For this review, take the finished solid that the model builds, in its own axes (mm). Face numbers are marked on the shaded views. Give positions to 0.01 mm unless a question says otherwise; leave off trailing zeros. Loops run counter-clockwise (first coordinate to the right, second up) from the corner with the lowest first, then second, coordinate; pieces in that order, holes last. Notation, with made-up numbers: (79.25, 2) - (101.25, 2) arc R23 ccw to (101.25, 27) - close; hole circle Ø5 at (58, 27). An arc over 180 degrees is marked (long way). Put each result on its own line as item: value.
from build123d import *

# Parameters (mm, degrees)
SKETCH1_W                = 28.4
SKETCH1_H                = 28.4
SKETCH1_W_2              = 25.4
SKETCH1_H_2              = 25.4
EXTRUDE_THIN1_DEPTH      = 400
SKETCH2_W                = 23
SKETCH2_H                = 23
SKETCH2_W_2              = 20
SKETCH2_H_2              = 20
EXTRUDE_THIN2_DEPTH      = 183
EXTRUDE_THIN2_DEPTH_BACK = 208.4
SKETCH3_W                = 60
SKETCH3_H                = 28.4
BOSS_EXTRUDE1_DEPTH      = 30
SKETCH4_W                = 23
SKETCH4_H                = 60
BOSS_EXTRUDE2_DEPTH      = 30
SKETCH5_R                = 5
BOSS_EXTRUDE3_DEPTH      = 30
SKETCH6_R                = 5
BOSS_EXTRUDE4_DEPTH      = 30
SKETCH7_R                = 5
BOSS_EXTRUDE5_DEPTH      = 30
SKETCH8_R                = 5
BOSS_EXTRUDE6_DEPTH      = 30
BOSS_EXTRUDE7_DEPTH      = 400
SKETCH10_W               = 372.349277715
SKETCH10_H               = 4
BOSS_EXTRUDE8_DEPTH      = 5
SKETCH24_R               = 30
BOSS_EXTRUDE20_DEPTH     = 10
SKETCH25_R               = 30
BOSS_EXTRUDE21_DEPTH     = 10
SKETCH26_R               = 30
BOSS_EXTRUDE22_DEPTH     = 10
SKETCH27_R               = 30
BOSS_EXTRUDE23_DEPTH     = 10
SKETCH28_W               = 18.859227369
SKETCH28_H               = 28.4
BOSS_EXTRUDE24_DEPTH     = 30
SKETCH29_R               = 3
BOSS_EXTRUDE25_DEPTH     = 276
SKETCH30_W               = 56.280454212
SKETCH30_H               = 13.197921903
BOSS_EXTRUDE26_DEPTH     = 40
SKETCH31_W               = 6.795939819
SKETCH31_H               = 6.783661409
BOSS_EXTRUDE27_DEPTH     = 20
SKETCH32_R               = 2.5
BOSS_EXTRUDE28_DEPTH     = 210
SKETCH33_W               = 5.188291065
SKETCH33_H               = 56.280454212
BOSS_EXTRUDE29_DEPTH     = 20
SKETCH34_W               = 21.924689073
SKETCH34_H               = 10.967349769
BOSS_EXTRUDE30_DEPTH     = 25
SKETCH35_R               = 3
BOSS_EXTRUDE31_DEPTH     = 20
SKETCH36_W               = 56.888194478
SKETCH36_H               = 11.912179608
BOSS_EXTRUDE32_DEPTH     = 5
SKETCH37_W               = 8
SKETCH37_H               = 8.77554695
BOSS_EXTRUDE33_DEPTH     = 10
SKETCH38_W               = 27.606480259
SKETCH38_H               = 24.3695053
SKETCH38_W_2             = 29.861732126
BOSS_EXTRUDE34_DEPTH     = 10
SKETCH39_W               = 14.536900962
SKETCH39_H               = 18.409696894
SKETCH39_W_2             = 14.264364069
SKETCH39_H_2             = 14.2
BOSS_EXTRUDE35_DEPTH     = 10


with BuildPart() as part:
    # Sketch1 → Extrude-Thin1 (new body)
    with BuildSketch(Plane(origin=(0, 0, 0), x_dir=(0, 0, -1), z_dir=(1, 0, 0))):
        Rectangle(SKETCH1_W, SKETCH1_H)
        Rectangle(SKETCH1_W_2, SKETCH1_H_2, mode=Mode.SUBTRACT)
    extrude(amount=EXTRUDE_THIN1_DEPTH)

    # Sketch2 → Extrude-Thin2 (add, two sides)
    with BuildSketch(Plane.XY.offset(14.2)) as extrude_thin2_sk:
        with Locations((200, -1.693644648)):
            Rectangle(SKETCH2_W, SKETCH2_H)
        with Locations((200, -1.693644648)):
            Rectangle(SKETCH2_W_2, SKETCH2_H_2, mode=Mode.SUBTRACT)
    extrude(amount=EXTRUDE_THIN2_DEPTH)
    extrude(extrude_thin2_sk.sketch, amount=-EXTRUDE_THIN2_DEPTH_BACK)

    # Sketch3 → Boss-Extrude1 (add)
    with BuildSketch(Plane(origin=(0, -14.2, 0), x_dir=(-1, 0, 0), z_dir=(0, -1, 0))):
        with Locations((-370, 0)):
            Rectangle(SKETCH3_W, SKETCH3_H)
        with Locations((-30, 0)):
            Rectangle(SKETCH3_W, SKETCH3_H)
    extrude(amount=BOSS_EXTRUDE1_DEPTH)

    # Sketch4 → Boss-Extrude2 (add)
    with BuildSketch(Plane(origin=(0, -13.193644648, 0), x_dir=(-1, 0, 0), z_dir=(0, -1, 0))):
        with Locations((-200, -167.2)):
            Rectangle(SKETCH4_W, SKETCH4_H)
        with Locations((-200, 164.2)):
            Rectangle(SKETCH4_W, SKETCH4_H)
    extrude(amount=BOSS_EXTRUDE2_DEPTH)

    # Sketch5 → Boss-Extrude3 (add)
    with BuildSketch(Plane(origin=(400, 0, 0), x_dir=(0, 0, -1), z_dir=(1, 0, 0))):
        with Locations((0, -34.2)):
            Circle(SKETCH5_R)
    extrude(amount=BOSS_EXTRUDE3_DEPTH)

    # Sketch6 → Boss-Extrude4 (add)
    with BuildSketch(Plane(origin=(0, 0, -194.2), x_dir=(-1, 0, 0), z_dir=(0, 0, -1))):
        with Locations((-200, -33.193644648)):
            Circle(SKETCH6_R)
    extrude(amount=BOSS_EXTRUDE4_DEPTH)

    # Sketch7 → Boss-Extrude5 (add)
    with BuildSketch(Plane.ZY):
        with Locations((0, -34.2)):
            Circle(SKETCH7_R)
    extrude(amount=BOSS_EXTRUDE5_DEPTH)

    # Sketch8 → Boss-Extrude6 (add)
    with BuildSketch(Plane.XY.offset(197.2)):
        with Locations((200, -33.193644648)):
            Circle(SKETCH8_R)
    extrude(amount=BOSS_EXTRUDE6_DEPTH)

    # Sketch9 → Boss-Extrude7 (add)
    with BuildSketch(Plane(origin=(0, 14.2, 0), x_dir=(1, 0, 0), z_dir=(0, 1, 0))):
        Polygon((10, 3.8), (20, 3.8), (20, 1.8), (13.177515759, 1.8), (13.177515759, -2.2), (20, -2.2), (20, -4.2), (10, -4.2), align=None)
        Polygon((380, 3.8), (390, 3.8), (390, -4.2), (380, -4.2), (380, -2.2), (385.526793474, -2.2), (385.526793474, 1.8), (380, 1.8), align=None)
    extrude(amount=BOSS_EXTRUDE7_DEPTH)

    # Sketch10 → Boss-Extrude8 (add)
    with BuildSketch(Plane(origin=(0, 264.2, 0), x_dir=(1, 0, 0), z_dir=(0, 1, 0))):
        with Locations((199.352154617, -0.2)):
            Rectangle(SKETCH10_W, SKETCH10_H)
    extrude(amount=BOSS_EXTRUDE8_DEPTH)

    # Sketch24 → Boss-Extrude20 (add)
    with BuildSketch(Plane(origin=(0, 0, -224.2), x_dir=(-1, 0, 0), z_dir=(0, 0, -1))):
        with Locations((-200, -33.193644648)):
            Circle(SKETCH24_R)
    extrude(amount=-BOSS_EXTRUDE20_DEPTH)

    # Sketch25 → Boss-Extrude21 (add)
    with BuildSketch(Plane.ZY.offset(30)):
        with Locations((0, -34.2)):
            Circle(SKETCH25_R)
    extrude(amount=-BOSS_EXTRUDE21_DEPTH)

    # Sketch26 → Boss-Extrude22 (add)
    with BuildSketch(Plane.XY.offset(227.2)):
        with Locations((200, -33.193644648)):
            Circle(SKETCH26_R)
    extrude(amount=-BOSS_EXTRUDE22_DEPTH)

    # Sketch27 → Boss-Extrude23 (add)
    with BuildSketch(Plane(origin=(430, 0, 0), x_dir=(0, 0, -1), z_dir=(1, 0, 0))):
        with Locations((0, -34.2)):
            Circle(SKETCH27_R)
    extrude(amount=-BOSS_EXTRUDE23_DEPTH)

    # Sketch28 → Boss-Extrude24 (add)
    with BuildSketch(Plane(origin=(0, 14.2, 0), x_dir=(1, 0, 0), z_dir=(0, 1, 0))):
        with Locations((262.964436909, 0)):
            Rectangle(SKETCH28_W, SKETCH28_H)
    extrude(amount=BOSS_EXTRUDE24_DEPTH)

    # Sketch29 → Boss-Extrude25 (add)
    with BuildSketch(Plane(origin=(0, 44.2, 0), x_dir=(1, 0, 0), z_dir=(0, 1, 0))):
        with Locations((262.978152894, 0)):
            Circle(SKETCH29_R)
    extrude(amount=BOSS_EXTRUDE25_DEPTH)

    # Sketch30 → Boss-Extrude26 (add)
    with BuildSketch(Plane(origin=(100, 0, 0), x_dir=(0, 0, -1), z_dir=(1, 0, 0))):
        with Locations((7.595285017, 269.051232914)):
            Rectangle(SKETCH30_W, SKETCH30_H)
    extrude(amount=BOSS_EXTRUDE26_DEPTH)

    # Sketch31 → Boss-Extrude27 (add)
    with BuildSketch(Plane(origin=(0, 264.2, 0), x_dir=(-1, 0, 0), z_dir=(0, -1, 0))):
        with Locations((-27.594001553, -0.077336563)):
            Rectangle(SKETCH31_W, SKETCH31_H)
    extrude(amount=BOSS_EXTRUDE27_DEPTH)

    # Sketch32 → Boss-Extrude28 (add)
    with BuildSketch(Plane(origin=(30.991971462, 0, 0), x_dir=(0, 0, -1), z_dir=(1, 0, 0))):
        with Locations((0, 256.564095002)):
            Circle(SKETCH32_R)
    extrude(amount=BOSS_EXTRUDE28_DEPTH)

    # Sketch33 → Boss-Extrude29 (add)
    with BuildSketch(Plane(origin=(0, 262.452271962, 0), x_dir=(-1, 0, 0), z_dir=(0, -1, 0))):
        with Locations((-121.53991064, 7.595285017)):
            Rectangle(SKETCH33_W, SKETCH33_H)
    extrude(amount=BOSS_EXTRUDE29_DEPTH)

    # Sketch34 → Boss-Extrude30 (add)
    with BuildSketch(Plane(origin=(0, 275.650193865, 0), x_dir=(1, 0, 0), z_dir=(0, 1, 0))):
        with Locations((120.531111369, 26.453283936)):
            Rectangle(SKETCH34_W, SKETCH34_H)
    extrude(amount=BOSS_EXTRUDE30_DEPTH)

    # Sketch35 → Boss-Extrude31 (add)
    with BuildSketch(Plane(origin=(0, 0, -31.93695882), x_dir=(-1, 0, 0), z_dir=(0, 0, -1))):
        with Locations((-119.378398528, 287.680723614)):
            Circle(SKETCH35_R)
    extrude(amount=BOSS_EXTRUDE31_DEPTH)

    # Sketch36 → Boss-Extrude32 (add)
    with BuildSketch(Plane(origin=(0, 0, -51.93695882), x_dir=(-1, 0, 0), z_dir=(0, 0, -1))):
        with Locations((-97.822495767, 288.961624672)):
            Rectangle(SKETCH36_W, SKETCH36_H)
    extrude(amount=BOSS_EXTRUDE32_DEPTH)

    # Sketch37 → Boss-Extrude33 (add)
    with BuildSketch(Plane.ZY.offset(-10)):
        with Locations((0.2, 409.812226525)):
            Rectangle(SKETCH37_W, SKETCH37_H)
    extrude(amount=BOSS_EXTRUDE33_DEPTH)

    # Sketch38 → Boss-Extrude34 (add)
    with BuildSketch(Plane.ZY.offset(-188.5)):
        with Locations((-180.396759871, -2.378397298)):
            Rectangle(SKETCH38_W, SKETCH38_H)
        with Locations((182.269133937, -2.378397298)):
            Rectangle(SKETCH38_W_2, SKETCH38_H)
    extrude(amount=BOSS_EXTRUDE34_DEPTH)

    # Sketch39 → Boss-Extrude35 (add)
    with BuildSketch(Plane(origin=(0, 0, -14.2), x_dir=(-1, 0, 0), z_dir=(0, 0, -1))):
        with Locations((-7.268450481, 4.995151553)):
            Rectangle(SKETCH39_W, SKETCH39_H)
        with Locations((-392.867817966, 7.1)):
            Rectangle(SKETCH39_W_2, SKETCH39_H_2)
    extrude(amount=BOSS_EXTRUDE35_DEPTH)


solid = part.part
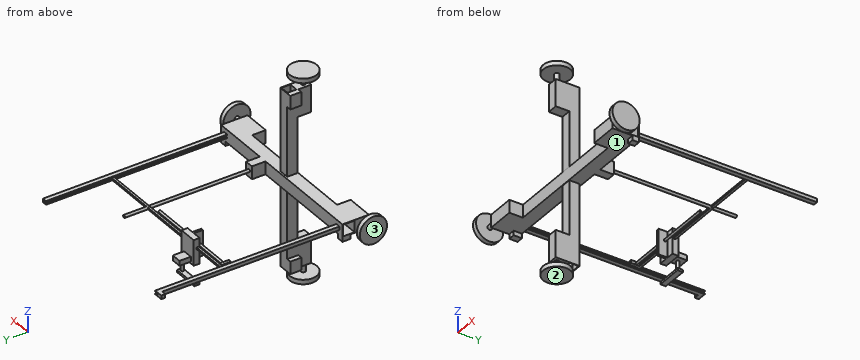
1) Take a section at A-A on x = 370. State the section outline as (y, z) points, and give its area (3 significant figures).
Geometry check:
outline: (-44.2, -14.2) - (14.2, -14.2) - (14.2, 14.2) - (-44.2, 14.2) - close; (264.2, -1.8) - (269.2, -1.8) - (269.2, 2.2) - (264.2, 2.2) - close; hole (-12.7, -12.7) - (12.7, -12.7) - (12.7, 12.7) - (-12.7, 12.7) - close
area: 1,030 mm²
2) Draft analysis for pull direction X (two halves, no side actions). For the marked faces 1, 2 and 3, state which applies: pulls with the +X half, pulls with the -X half, needs draft (parallel to the pull), parting line crosses it, or undercut.
Geometry check:
face 1: undercut
face 2: needs draft
face 3: pulls with the -X half
3) Take a section at C-C on y = 58. State the section outline as (x, z) points.
Geometry check:
outline: (10, -3.8) - (20, -3.8) - (20, -1.8) - (13.18, -1.8) - (13.18, 2.2) - (20, 2.2) - (20, 4.2) - (10, 4.2) - close; circle Ø6 at (262.98, 0); (380, -3.8) - (390, -3.8) - (390, 4.2) - (380, 4.2) - (380, 2.2) - (385.53, 2.2) - (385.53, -1.8) - (380, -1.8) - close
4) Take a section at B-B on y = 379. State the section outline as (x, z) points.
Geometry check:
outline: (10, -3.8) - (20, -3.8) - (20, -1.8) - (13.18, -1.8) - (13.18, 2.2) - (20, 2.2) - (20, 4.2) - (10, 4.2) - close; (380, -3.8) - (390, -3.8) - (390, 4.2) - (380, 4.2) - (380, 2.2) - (385.53, 2.2) - (385.53, -1.8) - (380, -1.8) - close
5) Insertion check: pin 1 Ø2 at (y, z) = (169.5, -2.5) entering from -X; pin 2 Ø1.5 at (x, y) = (59, 266.5) entering from +Z; pin 3 Ø1.5 at (y, z) = (8, 7) entering from +X. Each pin has a flat end and moves straight along its axis. Give the tip position at first contact, or say it passes through.
Geometry check:
pin 1: stops at x = 10
pin 2: stops at z = 2.2
pin 3: stops at x = 211.5
6) Wall thickness on line 1 (X direction, y = -11.5, z = 13); line 2 (Y direction, x = 207, z = 189); line 3 (X direction, y = -5.5, z = -57.5): over which ranges is each line inside the solid? List them lowest first.
Geometry check:
line 1: x = -30 to -20, 0 to 400, 420 to 430
line 2: y = -43.19 to -11.69, 8.31 to 9.81
line 3: x = 188.5 to 190, 210 to 211.5
7) Take a section at D-D on z = 41. State the section outline as (x, y) points.
Geometry check:
outline: (188.5, -13.19) - (211.5, -13.19) - (211.5, 9.81) - (188.5, 9.81) - close; hole (190, -11.69) - (210, -11.69) - (210, 8.31) - (190, 8.31) - close
